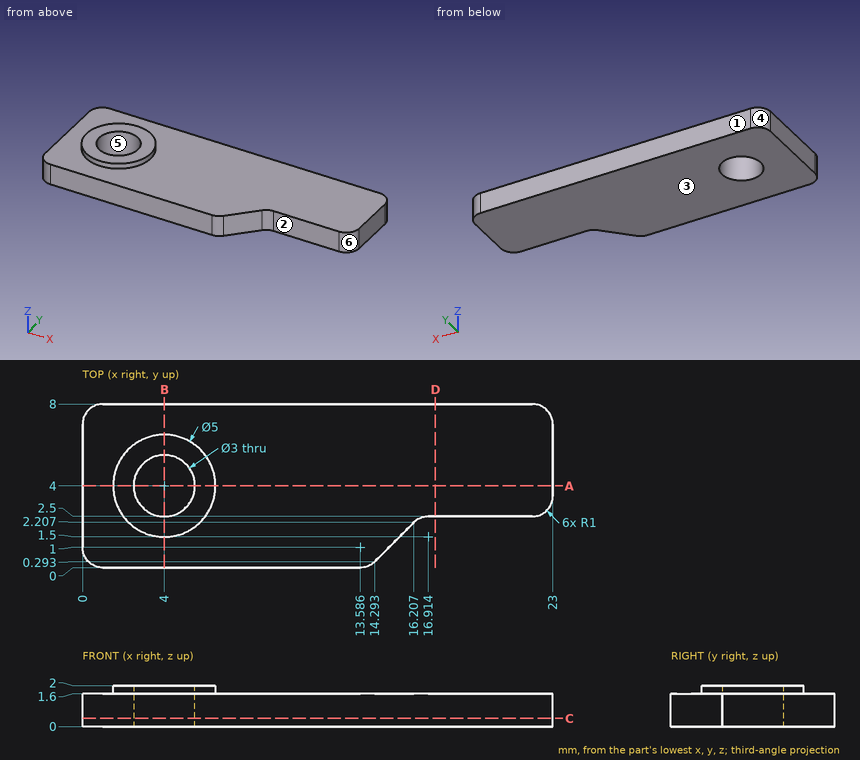
Can you work these out from the drawing? Everything is in mm from the part's minimum corner. A direction names the side the tool comes from. Give positions to 0.01 mm unless a question says otherwise; leave off trailing zeros. Order: outer loops, then holes, each group sorted by start corner. A loop starts at its lowest first (then second) coordinate and runs counter-clockwise, first axis right, second up. Notation, with made-up numbers: M 85.25,28 L 91.25,28 A14 ccw 91.25,33 Z; hole C -31.5,47.5 d1. An arc over 180 degrees is marked long. One line per question, with ' | ' between items.
1. I want a section at B-B (x = 4). List the corners of the cut face in (y, z) for me.
Results:
outline: M 0,0 L 2.5,0 L 2.5,2 L 1.5,2 L 1.5,1.6 L 0,1.6 Z; M 5.5,0 L 8,0 L 8,1.6 L 6.5,1.6 L 6.5,2 L 5.5,2 Z
2. I want a section at A-A (y = 4). List the corners of the cut face in (x, z) for me, and give its area (3 significant figures).
Results:
outline: M 0,0 L 2.5,0 L 2.5,2 L 1.5,2 L 1.5,1.6 L 0,1.6 Z; M 5.5,0 L 23,0 L 23,1.6 L 6.5,1.6 L 6.5,2 L 5.5,2 Z | area: 32.8 mm²
3. I want a section at D-D (x = 17.25). List the corners of the cut face in (y, z) for me.
Results:
outline: M 2.5,0 L 8,0 L 8,1.6 L 2.5,1.6 Z
4. I'm going to push flat-ended pins straight in: pin 1 (3.5 mm diameter, centred on x = 4, y = 4, fed in from +Z); pin 2 (2.5 mm diameter, centred on x = 12, y = 3.5, fed in from +Z). Where does each tip first touch, or does it pass through?
Results:
pin 1: z = 2 | pin 2: z = 1.6
5. For the marked faces 1 and 2, which set-ups out of +Z, -Z, +X, -X, +Y, -Y let a thin tool reach every point of the face, with its end or its side?
Results:
face 1: +Z, -Z, +X, -X, +Y | face 2: +Z, -Z, +X, -Y
6. If I drill on line 1 (Y direction, x = 4, z = 1.25); line 2 (Y direction, x = 17.5, z = 1.25); line 3 (Z direction, x = 14.5, y = 5.5), over which ranges is the centre line in solid material (lowest first)?
Results:
line 1: 0 to 2.5, 5.5 to 8 | line 2: 2.5 to 8 | line 3: 0 to 1.6
7. I want a section at C-C (z = 0.4). List the corners of the cut face in (x, y) for me, and give its area (3 significant figures).
Results:
outline: M 0,1 A1 ccw 1,0 L 13.59,0 A1 ccw 14.29,0.29 L 16.21,2.21 A1 cw 16.91,2.5 L 22,2.5 A1 ccw 23,3.5 L 23,7 A1 ccw 22,8 L 1,8 A1 ccw 0,7 Z; hole C 4,4 d3 | area: 157 mm²
8. We'd pull the mould along Y, two halves only. Please class the marked faces 3, 4, 5 and 6: +Y half, -Y half, draft (parallel to the pull), parting line (faces both ways), or undercut.
Results:
face 3: draft | face 4: +Y half | face 5: undercut | face 6: -Y half
